from build123d import *

# Parameters (mm, degrees)
SKETCH1_R           = 58.166
BOSS_EXTRUDE1_DEPTH = 21.971
SKETCH3_R           = 51.816
CUT_EXTRUDE2_DEPTH  = 18.796
CUT_EXTRUDE7_DEPTH  = 18.796
SKETCH8_R           = 58.166
BOSS_EXTRUDE4_DEPTH = 12.7
SKETCH9_R           = 6.477
CUT_EXTRUDE8_DEPTH  = 12.7


with BuildPart() as part:
    # Sketch1 → Boss-Extrude1 (new body)
    with BuildSketch(Plane(origin=(0, 0, 0), x_dir=(1, 0, 0), z_dir=(0, 1, 0))):
        Circle(SKETCH1_R)
    extrude(amount=BOSS_EXTRUDE1_DEPTH)

    # Sketch3 → Cut-Extrude2 (cut)
    with BuildSketch(Plane(origin=(0, 21.971, 0), x_dir=(1, 0, 0), z_dir=(0, 1, 0))):
        Circle(SKETCH3_R)
    extrude(amount=-CUT_EXTRUDE2_DEPTH, mode=Mode.SUBTRACT)

    # Sketch6 → Cut-Extrude7 (cut)
    with BuildSketch(Plane(origin=(0, 21.971, 0), x_dir=(1, 0, 0), z_dir=(0, 1, 0))):
        with BuildLine():
            Line((9.363048829, 50.963037318), (9.340756891, 57.411094892))
            ThreePointArc((9.340756891, 57.411094892), (2.903170649, 58.093503563), (-3.57037671, 58.056317194))
            Line((-3.57037671, 58.056317194), (-3.57037671, 51.692845406))
            ThreePointArc((-3.57037671, 51.692845406), (2.919232353, 51.733702153), (9.363048829, 50.963037318))
        make_face()
    extrude(amount=-CUT_EXTRUDE7_DEPTH, mode=Mode.SUBTRACT)

    # Sketch8 → Boss-Extrude4 (add)
    with BuildSketch(Plane.XZ):
        Circle(SKETCH8_R)
    extrude(amount=BOSS_EXTRUDE4_DEPTH)

    # Sketch9 → Cut-Extrude8 (cut)
    with BuildSketch(Plane.XZ.offset(12.7)):
        with Locations((-29.083, 0)):
            Circle(SKETCH9_R)
        with Locations((29.083, 0)):
            Circle(SKETCH9_R)
    extrude(amount=-CUT_EXTRUDE8_DEPTH, mode=Mode.SUBTRACT)


solid = part.part
CAD build for the part. Positions are in the model's coordinates, mm. A direction names the side the tool comes from. Give positions to 0.01 mm unless a question says otherwise; leave off trailing zeros. Write each loop counter-clockwise with the first axis right and the second up, starting at its lowest first coordinate (ties: lowest second). Pieces come first, ordered by that corner, then holes. Notation, with made-up numbers: (25.5, -38.75) - (60.5, -38.75) arc R27 cw to (60.5, -9.75) - close; hole circle Ø1 at (88, -39.5). An arc over 180 degrees is marked (long way). Put each result on its own line as item: value.
(1) Tool access for faces 5 (the cylindrical face through (-5.101, 12.705, 51.564)), 6 (the cylindrical face through (-34.223, -6.439, -3.941)), 7 (the flat face through (-1, -12.7, 1)), 8 (the flat face through (-3.57, 13, -55)): list every direction of +Z, -Z, +X, -X, +Y, -Y with a clear straight run to the whole face (end or side of a thin tool).
Working result:
face 5: +Y
face 6: -Y
face 7: +Z, -Z, +X, -X, -Y
face 8: -Z, +Y
(2) Wall check: L1, parallel to X at y = 17, z = 0; L2, parallel to Y at x = 1, z = 26.5 (3 decimals); L3, parallel to X at y = 5, z = -6. Give the ranges that are in metal, low to high.
Working result:
L1: -58.17 to -51.82, 51.82 to 58.17
L2: -12.7 to 3.175
L3: -57.86 to -51.47, 51.47 to 57.86
(3) Drop flat-ended pins along their axis: pin 1 Ø15 at (x, z) = (29.083, 0) entering from +Y (3 decimals); pin 2 Ø10 at (y, z) = (7, 7.5) entering from +X; pin 3 Ø4 at (x, z) = (-30.5, 2) entering from -Y. Give the stop position or say it passes through.
Working result:
pin 1: y = 3.175
pin 2: x = 58.11
pin 3: y = 0
(4) Saw through at C-C (x = -15). List the corners of the cut face in (y, z) (3 decimals), then the cut area to 3 significant figures.
Working result:
outline: (-12.7, -56.199) - (21.971, -56.199) - (21.971, -49.597) - (3.175, -49.597) - (3.175, 49.597) - (21.971, 49.597) - (21.971, 56.199) - (-12.7, 56.199) - close
area: 2,030 mm^2
(5) Saw through at D-D (y = 9). List the corners of the cut face in (x, z).
Working result:
outline: (-3.57, -58.06) - (-3.57, -51.69) arc R51.82 cw (long way) to (9.36, -50.96) - (9.34, -57.41) arc R58.17 ccw (long way) to start
(6) Saw through at B-B (y = -10). List the corners of the cut face in (x, z).
Working result:
outline: circle Ø116.33 at (0, 0); hole circle Ø12.95 at (-29.08, 0); hole circle Ø12.95 at (29.08, 0)
(7) Pull direction Z, two halves, no side cores. Call faces 1 (the flat face through (-1, 3.175, -4)), 2 (the cylindrical face through (22.612, -6.439, 0.285)), 3 (the cylindrical face through (-42.87, 4.88, 39.31)), 4 (the flat face through (-35, 21.971, 39)): released by +Z, released by -Z, zero draft, split by the parting line, or undercut.
Working result:
face 1: undercut
face 2: undercut
face 3: split by the parting line
face 4: zero draft
(8) Saw through at A-A (z = 0). List the corners of the cut face in (x, y) (3 decimals).
Working result:
outline: (-58.166, -12.7) - (-35.56, -12.7) - (-35.56, 0) - (-22.606, 0) - (-22.606, -12.7) - (22.606, -12.7) - (22.606, 0) - (35.56, 0) - (35.56, -12.7) - (58.166, -12.7) - (58.166, 21.971) - (51.816, 21.971) - (51.816, 3.175) - (-51.816, 3.175) - (-51.816, 21.971) - (-58.166, 21.971) - close
